```python
from build123d import *

# Parameters (mm, degrees)
F1_DEPTH = 1
F2_R     = 0.49999


# Not quite as in the source:
# - a fillet or chamfer is up to 0.001 mm smaller than in the source, because OpenCascade refuses the exact size


with BuildPart() as f1:
    # F0 (on Top) → F1 (new body)
    with BuildSketch(Plane.XY):
        with BuildLine():
            Line((16.6633232089, 47.1416340365), (-16.6633232089, 47.1416340365))
            ThreePointArc((-16.6633232089, 47.1416340365), (0, -50), (16.6633232089, 47.1416340365))
        make_face()
    extrude(amount=F1_DEPTH)

    # F2 (radius 0.5 in the source; OpenCascade refuses exactly that, so slightly less here)
    f2_edges = [f1.edges().sort_by_distance(p)[0] for p in [
        (0, 47.141634, 1),
        (0, -50, 1),
        (0, 47.141634, 0),
        (0, -50, 0),
    ]]
    fillet(f2_edges, radius=F2_R)


solid = f1.part
```
Geometry: final body of the model. Coordinates: model frame, mm. Coordinates: 2 decimals unless noted, no trailing zeros. Loops run counter-clockwise (first coordinate to the right, second up) from the corner with the lowest first, then second, coordinate; pieces in that order, holes last. Notation, with made-up numbers: (4.25, 52.5) -> (48.25, 52.5) arc R35 ccw to (48.25, 85.5) -> close; hole circle Ø6 at (47.25, 28). An arc over 180 degrees is marked (long way). Use a Markdown table: item, result. Add a question column.
(1) Pin query (flat end, axial travel): pin 1 Ø12 at (x, y) = (-30, -8) entering from -Z. Return the tip coordinate at first contact, or that it passes through.
(2) Section query A-A, the plane z = 0.7. Return loops of the section in (x, y), plus the area to 3 significant figures.
(3) Line query: line 1 along X through (y, z) = (-5.5, 0.9); line 2 along Y through (x, z) = (15.5, 0.75); line 3 along X through (y, z) = (-19, 0.9). Output: solid intervals per line, ascending.
Answer:
| question | item | result |
|---|---|---|
| 1 | pin 1 | stops at z = 0 |
| 2 | outline | (-16.66, 47.1) arc R49.96 ccw (long way) to (16.66, 47.1) -> close |
| 2 | area | 7,780 mm^2 |
| 3 | line 1 | x = -49.5 to 49.5 |
| 3 | line 2 | y = -47.47 to 47.07 |
| 3 | line 3 | x = -46.03 to 46.03 |
